```python
from build123d import *

# Parameters (mm, degrees)
SKETCH1_W           = 72
SKETCH1_H           = 65
SKETCH1_R           = 2.5
SKETCH1_R_2         = 1.6
BOSS_EXTRUDE1_DEPTH = 5
FILLET1_R           = 6
SKETCH2_W           = 15
SKETCH2_H           = 8
CUT_EXTRUDE1_DEPTH  = 2
CHAMFER1_SIZE       = 2
SKETCH3_W           = 0.5
SKETCH3_H           = 8
CUT_EXTRUDE2_DEPTH  = 0.5
CHAMFER2_SIZE       = 0.5
CHAMFER3_SIZE       = 0.25
CUT_EXTRUDE3_DEPTH  = 2.5


with BuildPart() as part:
    # Sketch1 → Boss-Extrude1 (new body)
    with BuildSketch(Plane(origin=(0, 0, 0), x_dir=(1, 0, 0), z_dir=(0, 1, 0))):
        with Locations((36, 32.5)):
            Rectangle(SKETCH1_W, SKETCH1_H)
        with Locations(Location((6, 6, 0), (0, 0, 270))):
            Circle(SKETCH1_R, mode=Mode.SUBTRACT)
        with Locations(Location((66, 6, 0), (0, 0, 90))):
            Circle(SKETCH1_R, mode=Mode.SUBTRACT)
        with Locations(Location((5, 49, 0), (0, 0, 270))):
            Circle(SKETCH1_R_2, mode=Mode.SUBTRACT)
        with Locations(Location((5, 35, 0), (0, 0, 270))):
            Circle(SKETCH1_R_2, mode=Mode.SUBTRACT)
        with Locations(Location((21, 39, 0), (0, 0, 270))):
            Circle(SKETCH1_R_2, mode=Mode.SUBTRACT)
        with Locations(Location((21, 59, 0), (0, 0, 270))):
            Circle(SKETCH1_R_2, mode=Mode.SUBTRACT)
        with Locations(Location((51, 59, 0), (0, 0, 270))):
            Circle(SKETCH1_R_2, mode=Mode.SUBTRACT)
        with Locations(Location((51, 39, 0), (0, 0, 270))):
            Circle(SKETCH1_R_2, mode=Mode.SUBTRACT)
        with Locations(Location((67, 29, 0), (0, 0, 270))):
            Circle(SKETCH1_R_2, mode=Mode.SUBTRACT)
        with Locations(Location((67, 15, 0), (0, 0, 270))):
            Circle(SKETCH1_R_2, mode=Mode.SUBTRACT)
        with Locations(Location((41, 6, 0), (0, 0, 270))):
            Circle(SKETCH1_R_2, mode=Mode.SUBTRACT)
        with Locations(Location((31, 6, 0), (0, 0, 270))):
            Circle(SKETCH1_R_2, mode=Mode.SUBTRACT)
        with BuildLine():
            Line((8.5, 59), (8.5, 57))
            ThreePointArc((8.5, 57), (6, 54.5), (3.5, 57))
            Line((3.5, 57), (3.5, 59))
            ThreePointArc((3.5, 59), (6, 61.5), (8.5, 59))
        make_face(mode=Mode.SUBTRACT)
        with BuildLine():
            Line((68.5, 59), (68.5, 57))
            ThreePointArc((68.5, 57), (66, 54.5), (63.5, 57))
            Line((63.5, 57), (63.5, 59))
            ThreePointArc((63.5, 59), (66, 61.5), (68.5, 59))
        make_face(mode=Mode.SUBTRACT)
    extrude(amount=BOSS_EXTRUDE1_DEPTH)

    # Fillet1
    fillet1_edges = [part.edges().sort_by_distance(p)[0] for p in [
        (0, 2.5, -65),
        (72, 2.5, -65),
        (72, 2.5, 0),
        (0, 2.5, 0),
    ]]
    fillet(fillet1_edges, radius=FILLET1_R)

    # Sketch2 → Cut-Extrude1 (cut)
    with BuildSketch(Plane(origin=(0, 5, 0), x_dir=(1, 0, 0), z_dir=(0, 1, 0))):
        with Locations((7.5, 42)):
            Rectangle(SKETCH2_W, SKETCH2_H)
        with Locations((64.5, 22)):
            Rectangle(SKETCH2_W, SKETCH2_H)
    extrude(amount=-CUT_EXTRUDE1_DEPTH, mode=Mode.SUBTRACT)

    # Chamfer1
    chamfer1_edges = [part.edges().sort_by_distance(p)[0] for p in [
        (57, 3, -22),
        (15, 3, -42),
    ]]
    chamfer(chamfer1_edges, length=CHAMFER1_SIZE - 0.0001)  # a hair under: the kernel refuses the full size

    # Sketch3 → Cut-Extrude2 (cut)
    with BuildSketch(Plane(origin=(0, 3, 0), x_dir=(1, 0, 0), z_dir=(0, 1, 0))):
        with Locations((1.5, 42)):
            Rectangle(SKETCH3_W, SKETCH3_H)
        with Locations((3.5, 42)):
            Rectangle(SKETCH3_W, SKETCH3_H)
        with Locations((5.5, 42)):
            Rectangle(SKETCH3_W, SKETCH3_H)
        with Locations((11.5, 42)):
            Rectangle(SKETCH3_W, SKETCH3_H)
        with Locations((7.5, 42)):
            Rectangle(SKETCH3_W, SKETCH3_H)
        with Locations((9.5, 42)):
            Rectangle(SKETCH3_W, SKETCH3_H)
        with Locations((70.5, 22)):
            Rectangle(SKETCH3_W, SKETCH3_H)
        with Locations((68.5, 22)):
            Rectangle(SKETCH3_W, SKETCH3_H)
        with Locations((66.5, 22)):
            Rectangle(SKETCH3_W, SKETCH3_H)
        with Locations((64.5, 22)):
            Rectangle(SKETCH3_W, SKETCH3_H)
        with Locations((62.5, 22)):
            Rectangle(SKETCH3_W, SKETCH3_H)
        with Locations((60.5, 22)):
            Rectangle(SKETCH3_W, SKETCH3_H)
    extrude(amount=-CUT_EXTRUDE2_DEPTH, mode=Mode.SUBTRACT)

    # Chamfer2
    chamfer2_edges = [part.edges().sort_by_distance(p)[0] for p in [
        (70.75, 3, -22),
        (70.25, 3, -22),
        (68.75, 3, -22),
        (68.25, 3, -22),
        (66.75, 3, -22),
        (66.25, 3, -22),
        (64.75, 3, -22),
        (64.25, 3, -22),
        (62.75, 3, -22),
        (62.25, 3, -22),
        (60.75, 3, -22),
        (60.25, 3, -22),
        (11.75, 3, -42),
        (11.25, 3, -42),
        (9.75, 3, -42),
        (9.25, 3, -42),
        (7.75, 3, -42),
        (7.25, 3, -42),
        (5.75, 3, -42),
        (5.25, 3, -42),
        (3.75, 3, -42),
        (3.25, 3, -42),
        (1.75, 3, -42),
        (1.25, 3, -42),
    ]]
    chamfer(chamfer2_edges, length=CHAMFER2_SIZE - 0.0001)  # a hair under: the kernel refuses the full size

    # Chamfer3
    chamfer3_edges = [part.edges().sort_by_distance(p)[0] for p in [
        (0, 3, -42),
        (72, 3, -22),
    ]]
    chamfer(chamfer3_edges, length=CHAMFER3_SIZE)

    # Sketch4 → Cut-Extrude3 (cut)
    with BuildSketch(Plane.XZ):
        Polygon((8.406366588, -49), (6.703183294, -46.05), (3.296816706, -46.05), (1.593633412, -49), (3.296816706, -51.95), (6.703183294, -51.95), align=None)
        Polygon((8.406366588, -35), (6.703183294, -32.05), (3.296816706, -32.05), (1.593633412, -35), (3.296816706, -37.95), (6.703183294, -37.95), align=None)
        Polygon((24.406366588, -39), (22.703183294, -36.05), (19.296816706, -36.05), (17.593633412, -39), (19.296816706, -41.95), (22.703183294, -41.95), align=None)
        Polygon((54.406366588, -39), (52.703183294, -36.05), (49.296816706, -36.05), (47.593633412, -39), (49.296816706, -41.95), (52.703183294, -41.95), align=None)
        Polygon((54.406366588, -59), (52.703183294, -56.05), (49.296816706, -56.05), (47.593633412, -59), (49.296816706, -61.95), (52.703183294, -61.95), align=None)
        Polygon((24.406366588, -59), (22.703183294, -56.05), (19.296816706, -56.05), (17.593633412, -59), (19.296816706, -61.95), (22.703183294, -61.95), align=None)
        Polygon((34.406366588, -6), (32.703183294, -3.05), (29.296816706, -3.05), (27.593633412, -6), (29.296816706, -8.95), (32.703183294, -8.95), align=None)
        Polygon((44.406366588, -6), (42.703183294, -3.05), (39.296816706, -3.05), (37.593633412, -6), (39.296816706, -8.95), (42.703183294, -8.95), align=None)
        Polygon((70.406366588, -15), (68.703183294, -12.05), (65.296816706, -12.05), (63.593633412, -15), (65.296816706, -17.95), (68.703183294, -17.95), align=None)
        Polygon((70.406366588, -29), (68.703183294, -26.05), (65.296816706, -26.05), (63.593633412, -29), (65.296816706, -31.95), (68.703183294, -31.95), align=None)
    extrude(amount=-CUT_EXTRUDE3_DEPTH, mode=Mode.SUBTRACT)


solid = part.part
```
Work out the finished part from the listing and answer in its coordinate system (mm). A direction names the side the tool comes from. Coordinates: 2 decimals unless noted, no trailing zeros. Order: outer loops, then holes, each group sorted by start corner. A loop starts at its lowest first (then second) coordinate and runs counter-clockwise, first axis right, second up. Notation, with made-up numbers: M 87,25.5 L 107,25.5 A35 ccw 107,58.5 Z; hole C -39,-36 d3. An arc over 180 degrees is marked long. Use CSV: the item, a comma, the result in double quotes.
1) Section A-A on x = 41 is taken. Write down the section's boundary in (y, z), plus the area to 3 significant figures.
Worked out:
outline,"M 0,-65 L 5,-65 L 5,-7.6 L 2.5,-7.6 L 2.5,-8.95 L 0,-8.95 Z; M 0,-3.05 L 2.5,-3.05 L 2.5,-4.4 L 5,-4.4 L 5,0 L 0,0 Z"
area,"302 mm^2"
2) For faces 1 (the face through (66.1, 2.5, -54.5)), 2 (the face through (41, 1, -3.05)), determine the directions among +Z, -Z, +X, -X, +Y, -Y from which every point of the face is accessible in a straight line to the end or side of a thin tool.
Worked out:
face 1,"+Y, -Y"
face 2,"-Y"
3) Section B-B on y = 1.65 is taken. Count the separate pieces of the cut face and the enclosed holes in it, plus the area to 3 significant figures.
Worked out:
separate pieces,"1"
enclosed holes,"14"
area,"4,250 mm^2"
4) Flat-ended cylindrical pins translate along their axes: pin 1 Ø2 at (x, y) = (4.5, 1.5) entering from +Z; pin 2 Ø0.8 at (x, y) = (67, 1.5) entering from -Z. Find the tip coordinate at first contact, or state that the pin passes through.
Worked out:
pin 1,"stops at z = -0.02"
pin 2,"stops at z = -64.97"
5) Determine the mould class of faces 3 (the face through (63.5, 2, -58)), 4 (the face through (52.5, 2.5, -37.6)) for opening direction Z: released by +Z, released by -Z, zero draft, split by the parting line, or undercut.
Worked out:
face 3,"undercut"
face 4,"undercut"
6) Section C-C on x = 48.5 is taken. Write down the section's boundary in (y, z), plus the area to 3 significant figures.
Worked out:
outline,"M 0,-65 L 5,-65 L 5,0 L 0,0 L 0,-37.43 L 2.5,-37.43 L 2.5,-40.57 L 0,-40.57 L 0,-57.43 L 2.5,-57.43 L 2.5,-60.57 L 0,-60.57 Z"
area,"309 mm^2"
7) Consider line 1 (Z direction, x = 21, y = 3.15); line 2 (Z direction, x = 22.5, y = 1); line 3 (X direction, y = 1.25, z = -33). Determine where each line is inside the solid, lowest interval first. Write a range as [from, to].
Worked out:
line 1,"z = [-65, -60.6], [-57.4, -40.6], [-37.4, 0]"
line 2,"z = [-65, -61.95], [-56.05, -41.95], [-36.05, 0]"
line 3,"x = [0, 2.75], [7.25, 72]"
